Check sheet for the modelled part. Datum: model origin and axes. Units: mm. A direction names the side the tool comes from. Round coordinates to 2 decimals unless told otherwise and drop trailing zeros. Order: outer loops, then holes, each group sorted by start corner. A loop starts at its lowest first (then second) coordinate and runs counter-clockwise, first axis right, second up.
from build123d import *

# Parameters (mm, degrees)
SKETCH012_W     = 600
SKETCH012_H     = 2200
PAD007_DEPTH    = 450
SKETCH010_W     = 540
SKETCH010_H     = 2160
POCKET002_DEPTH = 10
SKETCH011_W     = 2150
SKETCH011_H     = 815
POCKET003_DEPTH = 5


with BuildPart() as part:
    # Sketch012 → Pad007 (new body, symmetric)
    with BuildSketch(Plane.XZ):
        Rectangle(SKETCH012_W, SKETCH012_H)
    extrude(amount=PAD007_DEPTH, both=True)

    # Sketch010 (on Face6 of Pad007) → Pocket002 (cut)
    with BuildSketch(Plane.XZ.offset(450)):
        Rectangle(SKETCH010_W, SKETCH010_H)
    pocket002 = extrude(amount=-POCKET002_DEPTH, mode=Mode.SUBTRACT)

    # Mirrored: Pocket002 across XZ
    add(pocket002.mirror(Plane.XZ), mode=Mode.SUBTRACT)

    # Sketch011 (on Face3 of Mirrored) → Pocket003 (cut)
    with BuildSketch(Plane(origin=(300, 0, 0), x_dir=(0, 0, 1), z_dir=(1, 0, 0))):
        with Locations((-5, -2.5)):
            Rectangle(SKETCH011_W, SKETCH011_H)
    pocket003 = extrude(amount=-POCKET003_DEPTH, mode=Mode.SUBTRACT)

    # Mirrored001: Pocket003 across YZ
    add(pocket003.mirror(Plane.YZ), mode=Mode.SUBTRACT)


solid = part.part
1) Gauge pin test, flat ends, axial feed: pin 1 (6 mm diameter, centred on x = 65.5, z = 814.5, fed in from +Y); pin 2 (1.5 mm diameter, centred on y = -67, z = -239.5, fed in from -X); pin 3 (8 mm diameter, centred on x = -52, z = 76, fed in from -Y). Record the tip position at first contact, or that the pin passes through.
2) Sectioned sample at A-A on z = -35. Record the cut outline in (x, y).
3) Draft check along Y on faces 1 (the face through (295, -3, -20)), 2 (the face through (-290, -450, 5)), 3 (the face through (300, -435, -5)). Enter one of: pulls with the +Y half, pulls with the -Y half, needs draft (parallel to the pull), parting line crosses it, or undercut.
4) Set-up check for faces 4 (the face through (-4, 440, 15)), 5 (the face through (-4, -440, 15)), 6 (the face through (-295, -3, -20)), 7 (the face through (-4, -6, 1100)): record each of +Z, -Z, +X, -X, +Y, -Y from which the full face is reachable in a straight line by a thin tool's end or side.
5) Scan lines: line 1 (Y direction, x = 193.5, z = -237); line 2 (X direction, y = -350.5, z = 248.5). Record each from-to range of solid material in increasing order.
6) Sectioned sample at B-B on x = -50. Record the cut outline in (y, z), and give its area (3 significant figures).
7) Sectioned sample at C-C on y = 7. Record the cut outline in (x, z).
Values found:
1. pin 1: stops at y = 440
1. pin 2: stops at x = -295
1. pin 3: stops at y = -440
2. outline: (-300, -450) - (-270, -450) - (-270, -440) - (270, -440) - (270, -450) - (300, -450) - (300, -405) - (295, -405) - (295, 410) - (300, 410) - (300, 450) - (270, 450) - (270, 440) - (-270, 440) - (-270, 450) - (-300, 450) - (-300, 410) - (-295, 410) - (-295, -405) - (-300, -405) - close
3. face 1: undercut
3. face 2: pulls with the -Y half
3. face 3: needs draft
4. face 4: +Y
4. face 5: -Y
4. face 6: -X
4. face 7: +Z, +X, -X, +Y, -Y
5. line 1: y = -440 to 440
5. line 2: x = -295 to 295
6. outline: (-450, -1100) - (450, -1100) - (450, -1080) - (440, -1080) - (440, 1080) - (450, 1080) - (450, 1100) - (-450, 1100) - (-450, 1080) - (-440, 1080) - (-440, -1080) - (-450, -1080) - close
6. area: 1,940,000 mm2
7. outline: (-300, -1100) - (300, -1100) - (300, -1080) - (295, -1080) - (295, 1070) - (300, 1070) - (300, 1100) - (-300, 1100) - (-300, 1070) - (-295, 1070) - (-295, -1080) - (-300, -1080) - close
